Autodesk Inventor part; units mm, degrees
ref_plane "YZ Plane" through (0, 0, 0) normal (1, 0, 0) x (0, 1, 0)
ref_plane "XZ Plane" through (0, 0, 0) normal (0, 1, 0) x (-1, 0, 0)
ref_plane "XY Plane" through (0, 0, 0) normal (0, 0, 1) x (1, 0, 0)
sketch "Эскиз1" plane through (0, 0, 0) normal (0, 0, 1) x (1, 0, 0)
  arc A0 (0, 55) -> (0, -55) centre (0, 0) ccw
  line L0 (0, 55) -> (0, -55)
  dimension "d0" = 55
revolve "Вращение1" add sketch "Эскиз1" angle 360 about axis through (0, 55, 0) along (0, -1, 0)
sketch "Эскиз2" plane through (0, 0, 0) normal (1, 0, 0) x (0, 1, 0)
  line L0 (0, -10) -> (0, 10)
  line L1 (0, -10) -> (56, -10)
  line L2 (56, -10) -> (56, 10)
  line L3 (56, 10) -> (0, 10)
  point P0 (0, 0)
  point P1 (0, 0)
  dimension "d2" = 20
  dimension "d3" = 56
sketch "Эскиз3" plane through (0, 0, 0) normal (1, 0, 0) x (0, 1, 0)
  arc A0 (-325, 0) -> (-225, 0) centre (-275, 0) ccw
  line L0 (-225, 0) -> (-325, 0)
  point P0 (0, 0)
  dimension "d5" = 275
  dimension "d6" = 50
revolve "Вращение3" add sketch "Эскиз3" angle 180 about axis through (0, -225, 0) along (0, -1, 0)
sketch "Эскиз4" plane through (0, 0, 0) normal (0, 0, 1) x (1, 0, 0)
  line L0 (0, -325) -> (0, -225) construction
  line L1 (0, -325) -> (0, -225)
  line L2 (0, 5) -> (0, -225)
  arc A0 (49.749372, -280) -> (54.887665, 3.513433) centre (-1671.578894, -107) ccw
  line L3 (54.791865, 5) -> (0, 5) construction
  line L4 (49.749372, -280) -> (0, -280) construction
  arc A1 (0, -55) -> (54.887665, 3.513433) centre (0, 0) ccw
  arc A2 (49.749372, -280) -> (0, -225) centre (0, -275) ccw
  arc A3 (0, -325) -> (49.749372, -280) centre (0, -275) ccw construction
  arc A4 (0, -225) -> (0, -325) centre (0, -275) ccw construction
  arc A5 (54.772256, 5) -> (-54.772256, 5) centre (0, 0) ccw construction
  arc A6 (-54.772256, 5) -> (0, -55) centre (0, 0) ccw
  arc A7 (54.887665, 3.513433) -> (54.772256, 5) centre (0, 0) ccw construction
  point P0 (0, -128.982251)
  dimension "d10" = 5
  dimension "d11" = 110
  dimension "d12" = 5
revolve "Вращение4" add sketch "Эскиз4" angle 360 about axis through (0, 5, 0) along (0, -1, 0)
revolve "Вращение5" cut sketch "Эскиз2" angle 360 about axis through (0, 0, -10) along (0, 0, 1)
equation "\"d0\" = Shoulder_width"
equation "\"d11\" = 2 * Shoulder_width"
equation "\"shoulder_height\" = 275"
equation "\"Shoulder_width\" = 55"
properties part number "ч ASY human dummy 01"
Read the model definition and answer for the solid it produces. Units are mm, in the model's axes. Round coordinates to 2 decimals unless told otherwise and drop trailing zeros. Write each loop counter-clockwise with the first axis right and the second up, starting at its lowest first coordinate (ties: lowest second). Pieces come first, ordered by that corner, then holes.
1. Given pin 1 Ø2 at (x, z) = (-12, 13) entering from -Y; pin 2 Ø5 at (x, y) = (26, -228) entering from +Z; pin 3 Ø4 at (x, z) = (30, 10.5) entering from +Y, each flat-ended and moving along its own axis, determine where each tip first touches the part or whether it passes through.
2. Straight lines are drawn through the part: L1, parallel to X at y = -270, z = 21; L2, parallel to Z at x = -7.5, y = -197.5; L3, parallel to Z at x = -32.5, y = -265. For each, find the intervals that lie inside material, in ascending order.
3. The part is cut by section A-A, the plane y = -283.5. Determine the outline of the cut face in (x, z).
Values:
1. pin 1: stops at y = -228.63
1. pin 2: stops at z = 48.84
1. pin 3: stops at y = 46.23
2. L1: x = -46.17 to -45.1, 0 to 46.17
2. L2: z = -55.55 to 55.55
2. L3: z = -39.55 to -36.66, 36.66 to 39.55
3. outline: (0, -49.27) arc R49.27 ccw to (0, 49.27) - close
